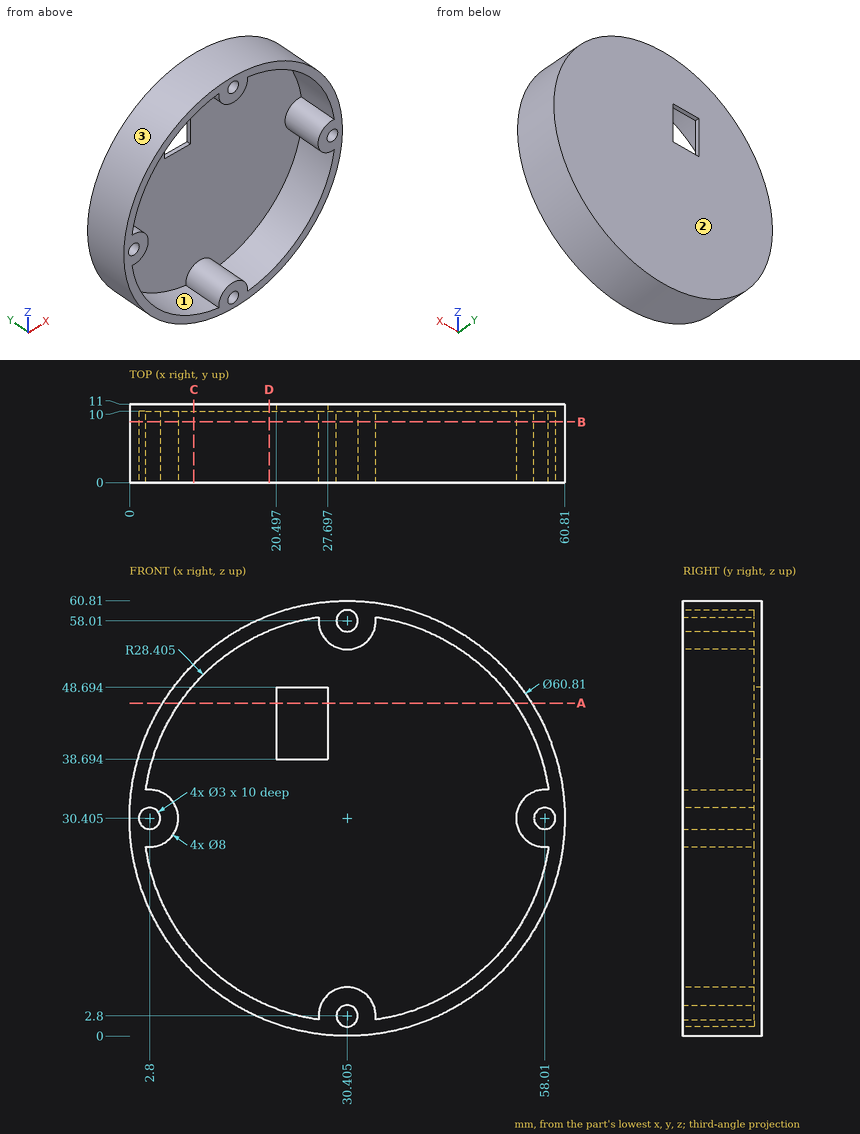
Geometry check sheet. Reference: drawing and pictorial views, mm from the part's lowest x, y, z. Round coordinates to 2 decimals unless told otherwise and drop trailing zeros. Write each loop counter-clockwise with the first axis right and the second up, starting at its lowest first coordinate (ties: lowest second). Pieces come first, ordered by that corner, then holes.
(1) Section check C-C (x = 9). Enter the section's corners in (y, z).
Returned:
outline: (0, 8.81) - (11, 8.81) - (11, 52) - (0, 52) - (0, 49.08) - (10, 49.08) - (10, 11.73) - (0, 11.73) - close
(2) Depth check by flat-ended pin: pin 1 Ø0.9 at (x, z) = (31, 3.5) entering from -Y; pin 2 Ø5 at (y, z) = (4, 26) entering from +X; pin 3 Ø0.5 at (y, z) = (10.5, 43) entering from -X; pin 4 Ø3.5 at (x, z) = (30.5, 58.5) entering from -Y. Enter the tip coordinate at first touch or a pass-through.
Returned:
pin 1: stops at y = 10
pin 2: stops at x = 60.75
pin 3: stops at x = 2.62
pin 4: stops at y = 0
(3) Section check B-B (y = 8.5). Enter the section's corners in (x, z) (1 decimal).
Returned:
outline: circle Ø60.8 at (30.4, 30.4); hole circle Ø3 at (2.8, 30.4); hole (2.3, 26.4) arc R28.4 ccw to (26.4, 2.3) arc R4 cw (long way) to (34.4, 2.3) arc R28.4 ccw to (58.5, 26.4) arc R4 cw (long way) to (58.5, 34.4) arc R28.4 ccw to (34.4, 58.5) arc R4 cw (long way) to (26.4, 58.5) arc R28.4 ccw to (2.3, 34.4) arc R4 cw (long way) to start; hole circle Ø3 at (30.4, 2.8); hole circle Ø3 at (30.4, 58); hole circle Ø3 at (58, 30.4)
(4) Material ranges on line 1 (Z direction, x = 30.5, y = 1.5); line 2 (X direction, y = 6.75, z = 55.5) (1 decimal); line 3 (Y direction, x = 40, z = 41.5), recorded low to high.
Returned:
line 1: z = 0 to 1.3, 4.3 to 6.8, 54.01 to 56.51, 59.51 to 60.81
line 2: x = 13.2 to 17.1, 27.3 to 33.5, 43.7 to 47.6
line 3: y = 10 to 11
(5) Section check A-A (z = 46.5). Enter the section's corners in (x, y).
Returned:
outline: (4.61, 0) - (7, 0) - (7, 10) - (20.5, 10) - (20.5, 11) - (4.61, 11) - close; (27.7, 10) - (53.81, 10) - (53.81, 0) - (56.2, 0) - (56.2, 11) - (27.7, 11) - close
(6) Section check D-D (x = 19.5). Enter the section's corners in (y, z).
Returned:
outline: (0, 2.02) - (11, 2.02) - (11, 58.79) - (0, 58.79) - (0, 56.63) - (10, 56.63) - (10, 4.18) - (0, 4.18) - close
(7) Mould release check, pull along X, two halves, no side actions. Record for the marked faces 1, 2 and 3: pulls with the +X half, pulls with the -X half, needs draft (parallel to the pull), parting line crosses it, or undercut.
Returned:
face 1: undercut
face 2: needs draft
face 3: parting line crosses it
